Model file for the job. Use its own axes, mm. Give positions to 0.01 mm unless a question says otherwise; leave off trailing zeros. Write each loop counter-clockwise with the first axis right and the second up, starting at its lowest first coordinate (ties: lowest second). Pieces come first, ordered by that corner, then holes. Notation, with made-up numbers: (16.5, 55.5) - (52.5, 55.5) arc R17 cw to (52.5, 62.5) - close; hole circle Ø6 at (87.5, 20). An arc over 180 degrees is marked (long way). One line per item, written item: value. Start each with the question number.
(1) Cut at C-C, the plane y = -1.25. List the corners of the cut face in (x, z).
(2) Cut at B-B, the plane x = 0. List the corners of the cut face in (y, z).
(3) Cut at A-A, the plane z = 0. List the corners of the cut face in (x, y), and give its area (3 significant figures).
(4) Probe L1, parallel to Z at x = 0, y = -2.3; L2, parallel to Z at x = 31.5, y = -4.7; L3, parallel to X at y = -1.4, z = -23. List the from-to ranges inside material, lowest first.
from build123d import *

# Parameters (mm, degrees)
F1_DEPTH = 5


with BuildPart() as f1:
    # F0 (on Front) → F1 (new body)
    with BuildSketch(Plane.XZ):
        Polygon((69.406778, -45), (69.406778, 0), (69.406778, 45), (-70.593222, 45), (-70.593222, -45), align=None)
        with BuildLine():
            ThreePointArc((-40, 0), (0, 40), (40, 0))
            ThreePointArc((40, 0), (0, -40), (-40, 0))
        make_face(mode=Mode.SUBTRACT)
    extrude(amount=F1_DEPTH)


solid = f1.part
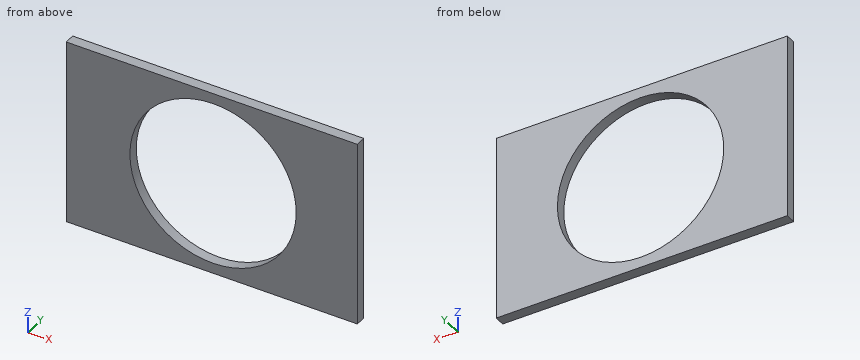
Answers follow:
1. outline: (-70.59, -45) - (69.41, -45) - (69.41, 45) - (-70.59, 45) - close; hole circle Ø80 at (0, 0)
2. outline: (-5, -45) - (0, -45) - (0, -40) - (-5, -40) - close; (-5, 40) - (0, 40) - (0, 45) - (-5, 45) - close
3. outline: (-70.59, -5) - (-40, -5) - (-40, 0) - (-70.59, 0) - close; (40, -5) - (69.41, -5) - (69.41, 0) - (40, 0) - close
3. area: 300 mm²
4. L1: z = -45 to -40, 40 to 45
4. L2: z = -45 to -24.65, 24.65 to 45
4. L3: x = -70.59 to -32.73, 32.73 to 69.41
